Check sheet for the modelled part. Datum: model origin and axes. Units: mm. A direction names the side the tool comes from. Coordinates: 2 decimals unless noted, no trailing zeros. Loops run counter-clockwise (first coordinate to the right, second up) from the corner with the lowest first, then second, coordinate; pieces in that order, holes last.
```python
from build123d import *

# Parameters (mm, degrees)
SKETCH_R     = 3.5
PAD_DEPTH    = 0.5
SKETCH001_R  = 2.5
PAD001_DEPTH = 8
SKETCH002_R  = 2.5
PAD002_DEPTH = 8


with BuildPart() as part:
    # Sketch → Pad (new body)
    with BuildSketch(Plane.YZ):
        Circle(SKETCH_R)
    extrude(amount=PAD_DEPTH)

    # Sketch001 (on Face3 of Pad) → Pad001 (join)
    with BuildSketch(Plane.YZ.offset(0.5)):
        Circle(SKETCH001_R)
    extrude(amount=PAD001_DEPTH)

    # Sketch002 (on Face2 of Pad001) → Pad002 (join)
    with BuildSketch(Plane(origin=(0, 0, 0), x_dir=(0, 1, 0), z_dir=(-1, 0, 0))):
        Circle(SKETCH002_R)
    extrude(amount=PAD002_DEPTH)


solid = part.part
```
1) Section check A-A on z = 0. Enter the section's corners in (x, y).
Answer sheet:
outline: (-8, -2.5) - (0, -2.5) - (0, -3.5) - (0.5, -3.5) - (0.5, -2.5) - (8.5, -2.5) - (8.5, 2.5) - (0.5, 2.5) - (0.5, 3.5) - (0, 3.5) - (0, 2.5) - (-8, 2.5) - close
2) Set-up check for faces 1 (the flat face through (-8, 0, 0)), 2 (the cylindrical face through (4.44, -0.54, -2.44)), 3 (the cylindrical face through (-3.94, -0.54, 2.44)): record each of +Z, -Z, +X, -X, +Y, -Y from which the full face is reachable in a straight line by a thin tool's end or side.
Answer sheet:
face 1: +Z, -Z, -X, +Y, -Y
face 2: +X
face 3: -X
3) Section check D-D on y = 2.75. Enter the section's corners in (x, z).
Answer sheet:
outline: (0, -2.17) - (0.5, -2.17) - (0.5, 2.17) - (0, 2.17) - close
4) Depth check by flat-ended pin: pin 1 (1.5 mm diameter, centred on x = -2.5, y = 0.5, fed in from +Z); pin 2 (1.5 mm diameter, centred on x = 6.5, z = 0, fed in from +Y). Enter the tip coordinate at first touch or a pass-through.
Answer sheet:
pin 1: stops at z = 2.5
pin 2: stops at y = 2.5
5) Scan lines: line 1 (X direction, y = -1.75, z = 3); line 2 (Y direction, x = -2, z = -1.75); line 3 (Y direction, x = -3.5, z = 0.5). Record each from-to range of solid material in increasing order.
Answer sheet:
line 1: x = 0 to 0.5
line 2: y = -1.79 to 1.79
line 3: y = -2.45 to 2.45
6) Section check C-C on x = -1.75. Enter the section's corners in (y, z), plus the area to 3 significant figures.
Answer sheet:
outline: circle Ø5 at (0, 0)
area: 19.6 mm2
